Source: CAD feature listing. Evaluate the final solid. Frame: model axes, mm. A direction names the side the tool comes from. Give positions to 0.01 mm unless a question says otherwise; leave off trailing zeros. Order: outer loops, then holes, each group sorted by start corner. A loop starts at its lowest first (then second) coordinate and runs counter-clockwise, first axis right, second up. Notation, with made-up numbers: (84.5, 59) - (95.5, 59) arc R26 cw to (95.5, 96) - close; hole circle Ø2 at (49.5, 23.5). An arc over 180 degrees is marked (long way). Write each question's results on one line, items separated by ' | '. Start each with the question number.
Item 1: Mould query, pull axis Z, two halves, no side actions, for faces 1 (the flat face through (20, -25, 0)), 2 (the flat face through (28, -48, 27)), 3 (the flat face through (5, -25, 40)). Classes: released by +Z, released by -Z, zero draft, split by the parting line, or undercut.
Item 2: Set-up query: faces 4 (the flat face through (45, -25, 30)), 5 (the flat face through (10, -49, 10)), 6 (the flat face through (0, -25, 15)), 7 (the flat face through (28, -49, 29.997)). Return all of +Z, -Z, +X, -X, +Y, -Y with unobstructed straight access to the full face (end or side cutting, diameter ignored); none if empty.
Item 3: Section D-D on z = 19. Output: boundary loops of the cut face in (x, y).
Item 4: Section C-C on y = -19.5. Output: boundary loops of the cut face in (x, z), and give its area (3 significant figures).
Item 5: Section B-B on x = 11. Output: boundary loops of the cut face in (y, z), and give its area (3 significant figures).
Item 6: Line query: line 1 along X through (y, z) = (-33.5, 21); line 2 along Y through (x, z) = (11, 11); line 3 along Z through (x, y) = (31.5, -23.5). Output: solid intervals per line, ascending.
Item 7: Section A-A on z = 5.5. Output: boundary loops of the cut face in (x, y), and give its area (3 significant figures).
Item 8: Contact query for flat-ended pins moving along their axis: pin 1 Ø1 at (x, y) = (28, -48.5) entering from +Z; pin 2 Ø5 at (y, z) = (-12.5, 21) entering from -X; pin 3 Ø1 at (y, z) = (-17, 31) entering from -X. Output: stop coordinate, or through.
```python
from build123d import *

# Parameters (mm, degrees)
PAD_DEPTH       = 50
SKETCH001_W     = 10
SKETCH001_H     = 20
POCKET_DEPTH    = 2
SKETCH002_W     = 3.446111
SKETCH002_H     = 6
SKETCH002_W_2   = 3.56074
SKETCH002_W_3   = 3.39247
SKETCH002_W_4   = 3.502147
POCKET001_DEPTH = 2


with BuildPart() as part:
    # Sketch → Pad (new body)
    with BuildSketch(Plane.XZ):
        Polygon((0, 0), (0, 30), (-10, 30), (20, 50), (50, 30), (40, 30), (40, 0), align=None)
    extrude(amount=PAD_DEPTH)

    # Sketch001 (on Face9 of Pad) → Pocket (cut)
    with BuildSketch(Plane.XZ.offset(50)):
        with Locations((15, 10)):
            Rectangle(SKETCH001_W, SKETCH001_H)
    extrude(amount=-POCKET_DEPTH, mode=Mode.SUBTRACT)

    # Sketch002 (on Face5 of Pocket) → Pocket001 (cut)
    with BuildSketch(Plane.XZ.offset(50)):
        with Locations((28.280043, 26.997097)):
            Rectangle(SKETCH002_W, SKETCH002_H)
        with Locations((33.783469, 26.997097)):
            Rectangle(SKETCH002_W_2, SKETCH002_H)
        with Locations((28.253223, 18.997097)):
            Rectangle(SKETCH002_W_3, SKETCH002_H)
        with Locations((33.700531, 18.997097)):
            Rectangle(SKETCH002_W_4, SKETCH002_H)
    extrude(amount=-POCKET001_DEPTH, mode=Mode.SUBTRACT)


solid = part.part
```
Evaluation:
1) face 1: released by -Z | face 2: undercut | face 3: released by +Z
2) face 4: -Z, +X, +Y, -Y | face 5: -Z, -Y | face 6: -Z, -X, +Y, -Y | face 7: -Y
3) outline: (0, -50) - (10, -50) - (10, -48) - (20, -48) - (20, -50) - (26.56, -50) - (26.56, -48) - (29.95, -48) - (29.95, -50) - (31.95, -50) - (31.95, -48) - (35.45, -48) - (35.45, -50) - (40, -50) - (40, 0) - (0, 0) - close
4) outline: (-10, 30) - (0, 30) - (0, 0) - (40, 0) - (40, 30) - (50, 30) - (20, 50) - close | area: 1,800 mm^2
5) outline: (-50, 20) - (-48, 20) - (-48, 0) - (0, 0) - (0, 44) - (-50, 44) - close | area: 2,160 mm^2
6) line 1: x = 0 to 40 | line 2: y = -48 to 0 | line 3: z = 0 to 42.33
7) outline: (0, -50) - (10, -50) - (10, -48) - (20, -48) - (20, -50) - (40, -50) - (40, 0) - (0, 0) - close | area: 1,980 mm^2
8) pin 1: stops at z = 45 | pin 2: stops at x = 0 | pin 3: stops at x = -9.25
